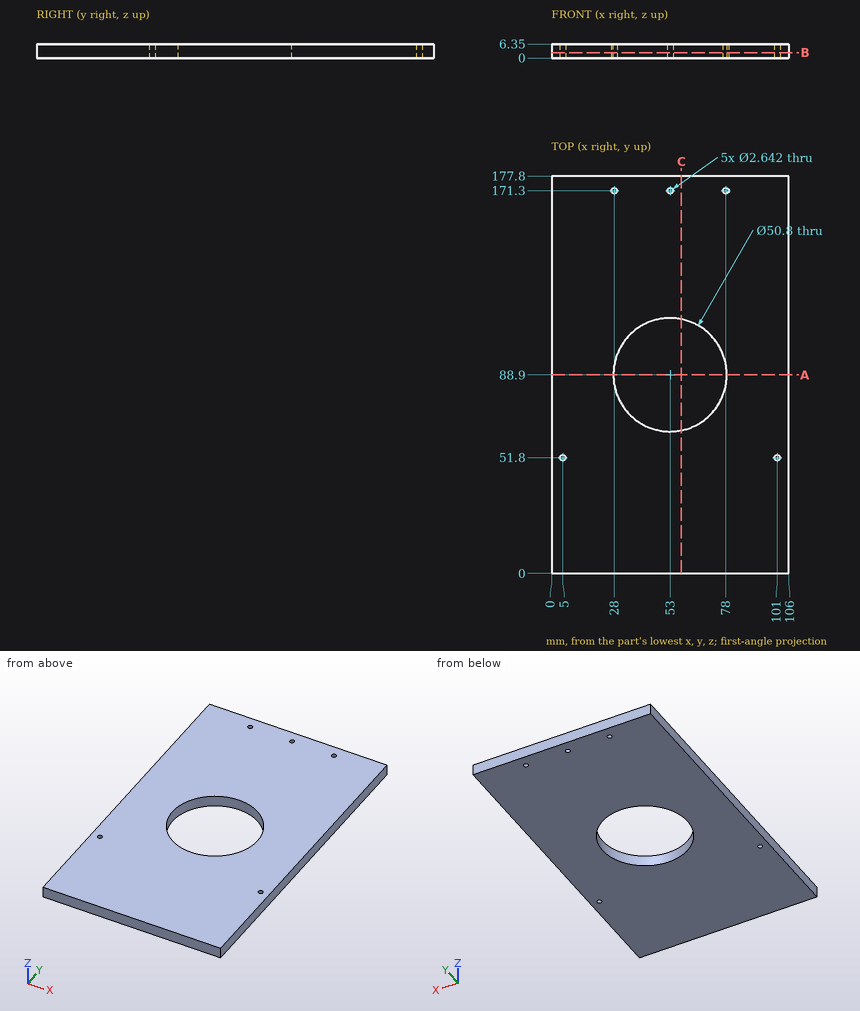
Input: dimensioned drawing with shaded views. Units: mm. Origin: part minimum x, y, z. Round coordinates to 2 decimals unless told otherwise and drop trailing zeros. Loops run counter-clockwise (first coordinate to the right, second up) from the corner with the lowest first, then second, coordinate; pieces in that order, holes last.
1) Material intervals for line 1 (X direction, y = 51.8, z = 3.5); line 2 (X direction, y = 87.5, z = 1.25); line 3 (Y direction, x = 53, z = 2.25), sorted ascending.
Ans:
line 1: x = 0 to 3.68, 6.32 to 99.68, 102.32 to 106
line 2: x = 0 to 27.64, 78.36 to 106
line 3: y = 0 to 63.5, 114.3 to 169.98, 172.62 to 177.8
2) Section query C-C on x = 58. Return the cut outline in (y, z).
Ans:
outline: (0, 0) - (64, 0) - (64, 6.35) - (0, 6.35) - close; (113.8, 0) - (177.8, 0) - (177.8, 6.35) - (113.8, 6.35) - close
3) Section query B-B on z = 2.5. Return the cut outline in (x, y), plus the area to 3 significant figures.
Ans:
outline: (0, 0) - (106, 0) - (106, 177.8) - (0, 177.8) - close; hole circle Ø2.64 at (5, 51.8); hole circle Ø2.64 at (28, 171.3); hole circle Ø50.8 at (53, 88.9); hole circle Ø2.64 at (53, 171.3); hole circle Ø2.64 at (78, 171.3); hole circle Ø2.64 at (101, 51.8)
area: 16,800 mm2
4) Section query A-A on y = 88.9. Return the cut outline in (x, z).
Ans:
outline: (0, 0) - (27.6, 0) - (27.6, 6.35) - (0, 6.35) - close; (78.4, 0) - (106, 0) - (106, 6.35) - (78.4, 6.35) - close
